```python
from build123d import *

# Parameters (mm, degrees)
SKETCH1_W                                           = 133.35
SKETCH1_H                                           = 31.75
BOSS_EXTRUDE1_DEPTH                                 = 12.7
CBORE_FOR_8_BINDING_HEAD_MACHINE_SCREW1_D           = 4.4958
CBORE_FOR_8_BINDING_HEAD_MACHINE_SCREW1_CBORE_D     = 9.525
CBORE_FOR_8_BINDING_HEAD_MACHINE_SCREW1_CBORE_DEPTH = 3.175
F_8_0_199_DIAMETER_HOLE1_D                          = 4.4958
SKETCH6_W                                           = 6.35
SKETCH6_H                                           = 9.525
BOSS_EXTRUDE2_DEPTH                                 = 25.4
F_8_0_199_DIAMETER_HOLE2_D                          = 4.4958
CBORE_FOR_6_BINDING_HEAD_MACHINE_SCREW1_D           = 3.7973
CBORE_FOR_6_BINDING_HEAD_MACHINE_SCREW1_CBORE_D     = 7.9375
CBORE_FOR_6_BINDING_HEAD_MACHINE_SCREW1_CBORE_DEPTH = 6.35
SKETCH12_R                                          = 2.286
CUT_EXTRUDE1_DEPTH                                  = 1.27
CUT_EXTRUDE2_START                                  = -6.35
SKETCH13_R                                          = 2.2479
CUT_EXTRUDE2_DEPTH                                  = 6.35
F_8_0_199_DIAMETER_HOLE3_D                          = 4.4958


with BuildPart() as part:
    # Sketch1 → Boss-Extrude1 (new body)
    with BuildSketch(Plane(origin=(0, 0, 0), x_dir=(1, 0, 0), z_dir=(0, 1, 0))):
        with Locations((66.675, 15.875)):
            Rectangle(SKETCH1_W, SKETCH1_H)
    extrude(amount=BOSS_EXTRUDE1_DEPTH)

    # CBORE for #8 Binding Head Machine Screw1 (through all)
    with Locations(Plane.XY):
        with Locations((6.35, 6.35), (127, 6.35)):
            CounterBoreHole(CBORE_FOR_8_BINDING_HEAD_MACHINE_SCREW1_D / 2, CBORE_FOR_8_BINDING_HEAD_MACHINE_SCREW1_CBORE_D / 2, CBORE_FOR_8_BINDING_HEAD_MACHINE_SCREW1_CBORE_DEPTH)

    # #8 (0.199) Diameter Hole1 (through all)
    with Locations(Plane(origin=(0, 12.7, 0), x_dir=(1, 0, 0), z_dir=(0, 1, 0))):
        with Locations((66.675, 12.954)):
            Hole(F_8_0_199_DIAMETER_HOLE1_D / 2)

    # Sketch6 → Boss-Extrude2 (add)
    with BuildSketch(Plane.XZ):
        with Locations((114.3, -12.954)):
            Rectangle(SKETCH6_W, SKETCH6_H)
        with Locations((19.05, -12.954)):
            Rectangle(SKETCH6_W, SKETCH6_H)
    extrude(amount=BOSS_EXTRUDE2_DEPTH)

    # #8 (0.199) Diameter Hole2 (through all)
    with Locations(Plane(origin=(117.475, 0, 0), x_dir=(0, 0, -1), z_dir=(1, 0, 0))):
        with Locations((12.954, -5.842), (12.954, -18.542)):
            Hole(F_8_0_199_DIAMETER_HOLE2_D / 2)

    # CBORE for #6 Binding Head Machine Screw1 (through all)
    with Locations(Plane(origin=(0, 0, 0), x_dir=(-1, 0, 0), z_dir=(0, -1, 0))):
        with Locations((-79.375, 12.954), (-92.075, 12.954)):
            CounterBoreHole(CBORE_FOR_6_BINDING_HEAD_MACHINE_SCREW1_D / 2, CBORE_FOR_6_BINDING_HEAD_MACHINE_SCREW1_CBORE_D / 2, CBORE_FOR_6_BINDING_HEAD_MACHINE_SCREW1_CBORE_DEPTH)

    # Sketch12 → Cut-Extrude1 (cut)
    with BuildSketch(Plane(origin=(0, 12.7, 0), x_dir=(1, 0, 0), z_dir=(0, 1, 0))):
        with Locations(Location((79.375, 12.954, 0), (0, 0, 270))):
            Circle(SKETCH12_R)
        with Locations(Location((92.075, 12.954, 0), (0, 0, 270))):
            Circle(SKETCH12_R)
    extrude(amount=-CUT_EXTRUDE1_DEPTH, mode=Mode.SUBTRACT)

    # Sketch13 → Cut-Extrude2 (cut)
    with BuildSketch(Plane(origin=(0, 12.7, 0), x_dir=(1, 0, 0), z_dir=(0, 1, 0)).offset(CUT_EXTRUDE2_START)):
        with Locations(Location((66.675, 12.954, 0), (0, 0, 270))):
            Circle(SKETCH13_R)
        Polygon((34.925, 6.604), (66.675, 6.604), (66.675, 12.954), (66.675, 19.304), (34.925, 19.304), align=None)
        Polygon((73.025, 6.604), (66.675, 6.604), (66.675, 12.954), (66.675, 19.304), (73.025, 19.304), align=None)
    extrude(amount=CUT_EXTRUDE2_DEPTH, mode=Mode.SUBTRACT)

    # #8 (0.199) Diameter Hole3 (through all)
    with Locations(Plane(origin=(0, 6.35, 0), x_dir=(1, 0, 0), z_dir=(0, 1, 0))):
        with Locations((53.975, 12.954), (41.275, 12.954)):
            Hole(F_8_0_199_DIAMETER_HOLE3_D / 2)


solid = part.part
```
Input: part model. Units: mm. Frame: model coordinates. A direction names the side the tool comes from. Round coordinates to 2 decimals unless told otherwise and drop trailing zeros. Loops run counter-clockwise (first coordinate to the right, second up) from the corner with the lowest first, then second, coordinate; pieces in that order, holes last. Notation, with made-up numbers: M -38,83 L 1,83 A24 ccw 1,115 Z; hole C 80.25,82.25 d1. An arc over 180 degrees is marked long. Answer in a Markdown table with one row per item. Add a question column.
1. Section D-D (x = 48). Output: boundary loops of the cut face in (y, z), and give its area (3 significant figures).
2. Contact query for flat-ended pins moving along their axis: pin 1 (4 mm diameter, centred on x = 59, z = -10.5, fed in from +Y); pin 2 (6 mm diameter, centred on y = -5.842, z = -12.954, fed in from +X) (3 decimals); pin 3 (5 mm diameter, centred on x = 92.075, z = -12.954, fed in from -Y); pin 4 (2.5 mm diameter, centred on y = -18.542, z = -12.954, fed in from -X). Output: stop coordinate, or through.
3. Section C-C (z = -22). Output: boundary loops of the cut face in (x, y), and give its area (3 significant figures).
4. Section A-A (y = -11.5). Output: boundary loops of the cut face in (x, z) (1 decimal), and give its area (3 significant figures).
5. Mould query, pull axis X, two halves, no side actions, for faces 4 (the face through (66, 6, -31.75)), 5 (the face through (90, 6.35, -14)), 6 (the face through (133.35, 6, -16)). Classes: released by +X, released by -X, zero draft, split by the parting line, or undercut.
6. Ray query, probe 1 along X at (y, z) = (6.5, -21); probe 2 along X at (y, z) = (8, -20.5); probe 3 along X at (y, z) = (7, -18) (3 decimals). Return the intervals inside material, ascending.
7. Set-up query: faces 1 (the face through (73.025, 9, -13)), 2 (the face through (114, -13, -17.716)), 3 (the face through (22.225, -13, -13)). Return all of +Z, -Z, +X, -X, +Y, -Y with unobstructed straight access to the full face (end or side cutting, diameter ignored); none if empty.
Values follow:
| question | item | result |
|---|---|---|
| 1 | outline | M 0,-31.75 L 12.7,-31.75 L 12.7,-19.3 L 6.35,-19.3 L 6.35,-6.6 L 12.7,-6.6 L 12.7,0 L 0,0 Z |
| 1 | area | 323 mm^2 |
| 2 | pin 1 | y = 6.35 |
| 2 | pin 2 | x = 117.475 |
| 2 | pin 3 | y = 6.35 |
| 2 | pin 4 | through |
| 3 | outline | M 0,0 L 133.35,0 L 133.35,12.7 L 0,12.7 Z; hole C 6.35,6.35 d4.5; hole C 127,6.35 d4.5 |
| 3 | area | 1,660 mm^2 |
| 4 | outline | M 15.9,-17.7 L 22.2,-17.7 L 22.2,-8.2 L 15.9,-8.2 Z; M 111.1,-17.7 L 117.5,-17.7 L 117.5,-8.2 L 111.1,-8.2 Z |
| 4 | area | 121 mm^2 |
| 5 | face 4 | zero draft |
| 5 | face 5 | undercut |
| 5 | face 6 | released by +X |
| 6 | probe 1 | 0 to 4.11, 8.59 to 124.76, 129.24 to 133.35 |
| 6 | probe 2 | 0 to 4.82, 7.88 to 125.47, 128.53 to 133.35 |
| 6 | probe 3 | 0 to 4.198, 8.502 to 34.925, 73.025 to 124.848, 129.152 to 133.35 |
| 7 | face 1 | +Y |
| 7 | face 2 | -Z, +X, -X, -Y |
| 7 | face 3 | +Z, -Z, -Y |
